Work out the finished part from the listing and answer in its coordinate system (mm). A direction names the side the tool comes from. Give positions to 0.01 mm unless a question says otherwise; leave off trailing zeros. Write each loop counter-clockwise with the first axis right and the second up, starting at its lowest first coordinate (ties: lowest second). Pieces come first, ordered by that corner, then holes.
1) Straight lines are drawn through the part: probe 1 along Z at (x, y) = (1.5, 1.35); probe 2 along X at (y, z) = (1.8, -2.5); probe 3 along Z at (x, y) = (7.35, 1.3). For each, find the intervals that lie inside material, in ascending order.
2) Given pin 1 Ø2 at (x, z) = (-6.5, -5.5) entering from +Y; pin 2 Ø1.5 at (x, z) = (-9, 0.5) entering from -Y; pin 3 Ø1.4 at (y, z) = (1, 0) entering from -X; pin 4 Ø2 at (x, z) = (-7.35, -5.7) entering from -Y, each flat-ended and moving along its own axis, determine where each tip first touches the part or whether it passes through.
3) Find section D-D (z = 2.25). Determine the outline of the cut face in (x, y).
4) Find section B-B (y = 2.45). Determine the outline of the cut face in (x, z).
5) Find section C-C (x = 3). Determine the outline of the cut face in (y, z), plus the area to 3 significant figures.
6) Determine the mould class of faces 4 (the face through (-5.5, 1, -7)), 5 (the face through (10.35, 3, 0)), 6 (the face through (-10.35, 3, 0)), 7 (the face through (0, 0, 6)) for opening direction X: pulls with the +X half, pulls with the -X half, needs draft (parallel to the pull), parting line crosses it, or undercut.
7) A tool of negligible diameter and unlimited length cuts with its end or side. For faces 1 (the face through (8, 2.8, 0)), 2 (the face through (8.824, 4.113, 7.052)), 3 (the face through (-8, 2.8, 0)), from which of +Z, -Z, +X, -X, +Y, -Y can it reach the whole face along a straight path? Write none if from no direction.
8) Find section A-A (y = 0.95). Determine the outline of the cut face in (x, z), plus the area to 3 significant figures.
```python
from build123d import *

# Parameters (mm, degrees)
F0_W           = 20.7
F0_H           = 17.4
F1_DEPTH       = 5
F2_W           = 11.5
F2_H           = 11.5
F3_DEPTH       = 2.8
F5_R           = 1
F7_DEPTH       = 2.8
F9_D           = 2.5
F9_DEPTH       = 5
F9_CBORE_D     = 4
F9_CBORE_DEPTH = 1.8
F9_TIP         = 0.7510757738
F11_DEPTH      = 2


# Not quite as in the source:
# - a feature names something its author has since deleted; it is built from what else it names


with BuildPart() as f1:
    # F0 (on Front) → F1 (new body)
    with BuildSketch(Plane.XZ):
        Rectangle(F0_W, F0_H)
    extrude(amount=-F1_DEPTH)

    # F2 (on face) → F3 (cut)
    with BuildSketch(Plane.XZ):
        Rectangle(F2_W, F2_H)
    extrude(amount=-F3_DEPTH, mode=Mode.SUBTRACT)

    # F5
    f5_edges = [f1.edges().sort_by_distance(p)[0] for p in [
        (-5.75, 1.4, 5.75),
        (5.75, 1.4, 5.75),
        (-5.75, 1.4, -5.75),
        (5.75, 1.4, -5.75),
    ]]
    fillet(f5_edges, radius=F5_R)

    # F6 (on face) → F7 (cut)
    with BuildSketch(Plane.XZ):
        with BuildLine():
            Line((-10.35, -1.5), (-8, -1.5))
            ThreePointArc((-8, -1.5), (-6.5, 0), (-8, 1.5))
            Line((-8, 1.5), (-10.35, 1.5))
            Line((-10.35, 1.5), (-10.35, -1.5))
        make_face()
        with BuildLine():
            ThreePointArc((8, 1.5), (6.5, 0), (8, -1.5))
            Line((8, -1.5), (8, 0))
            Line((8, 0), (8, 1.5))
        make_face()
        Polygon((8, -1.5), (10.35, -1.5), (10.35, 1.5), (8, 1.5), (8, 0), align=None)
    extrude(amount=-F7_DEPTH, mode=Mode.SUBTRACT)

    # F9
    with Locations(Plane(origin=(0, 5, 0), x_dir=(-1, 0, 0), z_dir=(0, 1, 0))):
        with Locations((7.35, -5.7), (-7.35, 5.7)):
            CounterBoreHole(F9_D / 2, F9_CBORE_D / 2, F9_CBORE_DEPTH, depth=F9_DEPTH)
            with Locations((0, 0, -(F9_DEPTH + F9_TIP / 2))):  # 118° drill point
                Cone(0, F9_D / 2, F9_TIP, mode=Mode.SUBTRACT)

    # F10 (on face) → F11 (cut)
    with BuildSketch(Plane.XZ):
        with BuildLine():
            Line((4.75, -5.75), (2.5, -5.75))
            Line((2.5, -5.75), (2.5, -8.7))
            Line((2.5, -8.7), (5.5, -8.7))
            Line((5.5, -8.7), (5.5, -5.4114378278))
            ThreePointArc((5.5, -5.4114378278), (5.1614378278, -5.6614378278), (4.75, -5.75))
        make_face()
        with BuildLine():
            Line((-2.5, -5.75), (-4.75, -5.75))
            ThreePointArc((-4.75, -5.75), (-5.1614378278, -5.6614378278), (-5.5, -5.4114378278))
            Line((-5.5, -5.4114378278), (-5.5, -8.7))
            Line((-5.5, -8.7), (-2.5, -8.7))
            Line((-2.5, -8.7), (-2.5, -5.75))
        make_face()
    extrude(amount=-F11_DEPTH, mode=Mode.SUBTRACT)


solid = f1.part
```
Results:
1. probe 1: z = -8.7 to -5.75, 5.75 to 8.7
1. probe 2: x = -10.35 to -5.75, 5.75 to 10.35
1. probe 3: z = -8.7 to -1.35, 1.35 to 4.45, 6.95 to 8.7
2. pin 1: stops at y = 3.2
2. pin 2: stops at y = 2.8
2. pin 3: stops at x = -6.67
2. pin 4: passes through
3. outline: (-10.35, 0) - (-5.75, 0) - (-5.75, 2.8) - (5.75, 2.8) - (5.75, 0) - (10.35, 0) - (10.35, 5) - (-10.35, 5) - close
4. outline: (-10.35, -8.7) - (10.35, -8.7) - (10.35, -1.5) - (8, -1.5) arc R1.5 cw to (8, 1.5) - (10.35, 1.5) - (10.35, 8.7) - (-10.35, 8.7) - (-10.35, 1.5) - (-8, 1.5) arc R1.5 cw to (-8, -1.5) - (-10.35, -1.5) - close; hole circle Ø2.5 at (-7.35, -5.7); hole (-5.75, -4.75) arc R1 ccw to (-4.75, -5.75) - (4.75, -5.75) arc R1 ccw to (5.75, -4.75) - (5.75, 4.75) arc R1 ccw to (4.75, 5.75) - (-4.75, 5.75) arc R1 ccw to (-5.75, 4.75) - close; hole circle Ø2.5 at (7.35, 5.7)
5. outline: (0, 5.75) - (2.8, 5.75) - (2.8, -5.75) - (2, -5.75) - (2, -8.7) - (5, -8.7) - (5, 8.7) - (0, 8.7) - close
5. area: 48.9 mm2
6. face 4: undercut
6. face 5: pulls with the +X half
6. face 6: pulls with the -X half
6. face 7: needs draft
7. face 1: +X, -Y
7. face 2: +Y
7. face 3: -X, -Y
8. outline: (-10.35, -8.7) - (-5.5, -8.7) - (-5.5, -5.41) arc R1 cw to (-5.75, -4.75) - (-5.75, 4.75) arc R1 cw to (-4.75, 5.75) - (4.75, 5.75) arc R1 cw to (5.75, 4.75) - (5.75, -4.75) arc R1 cw to (5.5, -5.41) - (5.5, -8.7) - (10.35, -8.7) - (10.35, -1.5) - (8, -1.5) arc R1.5 cw to (8, 1.5) - (10.35, 1.5) - (10.35, 8.7) - (-10.35, 8.7) - (-10.35, 1.5) - (-8, 1.5) arc R1.5 cw to (-8, -1.5) - (-10.35, -1.5) - close; (-2.5, -8.7) - (2.5, -8.7) - (2.5, -5.75) - (-2.5, -5.75) - close; hole circle Ø2.5 at (-7.35, -5.7); hole circle Ø2.5 at (7.35, 5.7)
8. area: 180 mm2
